from build123d import *

# Parameters (mm, degrees)
SKETCH1_W           = 20.6
SKETCH1_H           = 14.3
SKETCH1_R           = 1.6
BOSS_EXTRUDE1_DEPTH = 1.6
SKETCH2_W           = 18.658076696
SKETCH2_H           = 2.368570216
BOSS_EXTRUDE2_DEPTH = 9


with BuildPart() as part:
    # Sketch1 → Boss-Extrude1 (new body)
    with BuildSketch(Plane(origin=(0, 0, 0), x_dir=(1, 0, 0), z_dir=(0, 1, 0))):
        Rectangle(SKETCH1_W, SKETCH1_H)
        with Locations((-7.5, 4.95)):
            Circle(SKETCH1_R, mode=Mode.SUBTRACT)
        with Locations((7.5, 4.95)):
            Circle(SKETCH1_R, mode=Mode.SUBTRACT)
    extrude(amount=BOSS_EXTRUDE1_DEPTH)

    # Sketch2 → Boss-Extrude2 (add)
    with BuildSketch(Plane(origin=(0, 1.6, 0), x_dir=(1, 0, 0), z_dir=(0, 1, 0))):
        with Locations((0, -5.731493021)):
            Rectangle(SKETCH2_W, SKETCH2_H)
    extrude(amount=BOSS_EXTRUDE2_DEPTH)


solid = part.part
The model under review builds one solid part; all positions refer to its coordinate system, in mm. A direction names the side the tool comes from. Round coordinates to 2 decimals unless told otherwise and drop trailing zeros. Write each loop counter-clockwise with the first axis right and the second up, starting at its lowest first coordinate (ties: lowest second). Pieces come first, ordered by that corner, then holes. Notation, with made-up numbers: M -32.75,60 L 5.25,60 A20 cw 5.25,71 Z; hole C 15.5,49 d4. An arc over 180 degrees is marked long. Use a Markdown table: item, result. Add a question column.
Q1. We need section A-A, the plane x = 7.5. State the section outline as (y, z) points.
Q2. To check wall thickness, follow line 1 (X direction, y = 0.8, z = -4.95); line 2 (Z direction, x = -7.5, y = 1); line 3 (Y direction, x = -6, z = 1.25). State the ranges of each line that lie inside material, in increasing order.
Q3. The part is to be moulded in two halves that separate along Z. For faces 1 (the face through (0, 6, 4.547)), 2 (the face through (-7.708, 0.789, -6.536)), 3 (the face through (10.3, 1, 0)), 4 (the face through (6.32, 0.79, -6.03)), say which applies: pulls with the +Z half, pulls with the -Z half, needs draft (parallel to the pull), parting line crosses it, or undercut.
Q4. We need section C-C, the plane x = 3.25. State the section outline as (y, z) points.
Q5. We need section B-B, the plane z = -4.95. State the section outline as (x, y) points.
Q6. Insertion check: pin 1 (2.5 mm diameter, centred on x = 0.5, y = 6.5, fed in from +Z); pin 2 (1.2 mm diameter, centred on y = 7, z = 6, fed in from -X); pin 3 (4.5 mm diameter, centred on x = 0.5, z = -3, fed in from +Y). Each pin has a flat end and moves straight along its axis. Give the tip position at first contact, or say it passes through.
Q7. Machinability: for faces 5 (the face through (9.329, 6, 6)), 6 (the face through (0, 6, 6.916)), 7 (the face through (-9.329, 6, 6)), which of the approach directions +Z, -Z, +X, -X, +Y, -Y give a long, thin tool a straight path to every point of the face, cutting with its end or side? Answer none if there is none.
Q8. We need section D-D, the plane y = 0.75. State the section outline as (x, z) points, plus the area to 3 significant figures.
Findings below:
| question | item | result |
|---|---|---|
| 1 | outline | M 0,-7.15 L 1.6,-7.15 L 1.6,-6.55 L 0,-6.55 Z; M 0,-3.35 L 1.6,-3.35 L 1.6,4.55 L 10.6,4.55 L 10.6,6.92 L 1.6,6.92 L 1.6,7.15 L 0,7.15 Z |
| 2 | line 1 | x = -10.3 to -9.1, -5.9 to 5.9, 9.1 to 10.3 |
| 2 | line 2 | z = -7.15 to -6.55, -3.35 to 7.15 |
| 2 | line 3 | y = 0 to 1.6 |
| 3 | face 1 | pulls with the -Z half |
| 3 | face 2 | undercut |
| 3 | face 3 | needs draft |
| 3 | face 4 | undercut |
| 4 | outline | M 0,-7.15 L 1.6,-7.15 L 1.6,4.55 L 10.6,4.55 L 10.6,6.92 L 1.6,6.92 L 1.6,7.15 L 0,7.15 Z |
| 5 | outline | M -10.3,0 L -9.1,0 L -9.1,1.6 L -10.3,1.6 Z; M -5.9,0 L 5.9,0 L 5.9,1.6 L -5.9,1.6 Z; M 9.1,0 L 10.3,0 L 10.3,1.6 L 9.1,1.6 Z |
| 6 | pin 1 | stops at z = 6.92 |
| 6 | pin 2 | stops at x = -9.33 |
| 6 | pin 3 | stops at y = 1.6 |
| 7 | face 5 | +Z, -Z, +X, +Y |
| 7 | face 6 | +Z, +X, -X, +Y |
| 7 | face 7 | +Z, -Z, -X, +Y |
| 8 | outline | M -10.3,-7.15 L 10.3,-7.15 L 10.3,7.15 L -10.3,7.15 Z; hole C -7.5,-4.95 d3.2; hole C 7.5,-4.95 d3.2 |
| 8 | area | 278 mm² |
